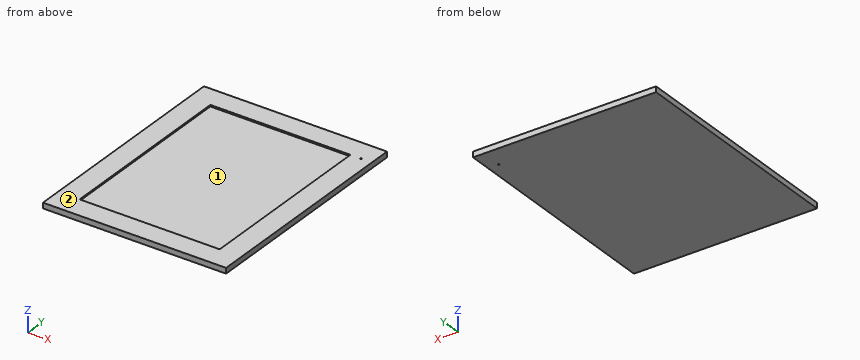
from build123d import *

# Parameters (mm, degrees)
SKETCH1_W          = 596
SKETCH1_H          = 746
DOOR_PART_DEPTH    = 18
SKETCH6_R          = 2.5
BASE_SINGLE_DEPTH  = 956.016230229
SKETCH7_W          = 456
SKETCH7_H          = 606
CUT_EXTRUDE1_DEPTH = 5


with BuildPart() as part:
    # Sketch1 → Door Part (new body)
    with BuildSketch(Plane.XY):
        with Locations((-298, -373)):
            Rectangle(SKETCH1_W, SKETCH1_H)
    extrude(amount=-DOOR_PART_DEPTH)

    # Sketch6 → Base Single (cut, through all)
    with BuildSketch(Plane.XY):
        with Locations((-35, -70)):
            Circle(SKETCH6_R)
    extrude(amount=-BASE_SINGLE_DEPTH, mode=Mode.SUBTRACT)

    # Sketch7 → Cut-Extrude1 (cut)
    with BuildSketch(Plane.XY):
        with Locations((-298, -373)):
            Rectangle(SKETCH7_W, SKETCH7_H)
    extrude(amount=-CUT_EXTRUDE1_DEPTH, mode=Mode.SUBTRACT)


solid = part.part
For this review, take the finished solid that the model builds, in its own axes (mm). Face numbers are marked on the shaded views. Round coordinates to 2 decimals unless told otherwise and drop trailing zeros. Order: outer loops, then holes, each group sorted by start corner. A loop starts at its lowest first (then second) coordinate and runs counter-clockwise, first axis right, second up. Notation, with made-up numbers: (21.25, -23.5) -> (40.25, -23.5) arc R18 ccw to (40.25, -16.5) -> close; hole circle Ø4 at (-6, 68). An arc over 180 degrees is marked (long way). Write item = value, one per line. Start each with the question number.
1) Insertion check: pin 1 (5 mm diameter, centred on x = -130.5, y = -143, fed in from +Z). The pin has a flat end and moves straight along its axis. Give the tip position at first contact, or say it passes through.
2) Take a section at A-A on y = -660.5. State the section outline as (x, z) points.
3) Take a section at B-B on x = -218. State the section outline as (y, z) points.
4) To check wall thickness, follow line 1 (Y direction, x = -35, z = -9.5); line 2 (Y direction, x = -409, z = -3.75); line 3 (X direction, y = -131.5, z = -4.5). State the ranges of each line that lie inside material, in increasing order. Write a range as from..to.
5) The part is to be moulded in two halves that separate along Y. For the marked faces 1 and 2, say which applies: +Y half, -Y half, draft (parallel to the pull), parting line (faces both ways), or undercut.
Verdict:
q1.pin_1 = -5
q2.outline = (-596, -18) -> (0, -18) -> (0, 0) -> (-70, 0) -> (-70, -5) -> (-526, -5) -> (-526, 0) -> (-596, 0) -> close
q3.outline = (-746, -18) -> (0, -18) -> (0, 0) -> (-70, 0) -> (-70, -5) -> (-676, -5) -> (-676, 0) -> (-746, 0) -> close
q4.line_1 = -746..-72.5, -67.5..0
q4.line_2 = -746..-676, -70..0
q4.line_3 = -596..-526, -70..0
q5.face_1 = undercut
q5.face_2 = draft
